```python
from build123d import *


with BuildPart() as f1:
    # F0 (on Front) → F1 (revolve)
    with BuildSketch(Plane.XZ):
        with BuildLine():
            Line((15.425971, 19.134293), (16, 0))
            Line((16, 0), (19, 0))
            Line((19, 0), (19.371627, 18.581355))
            ThreePointArc((19.371627, 18.581355), (19.209023, 19.949907), (18.678973, 21.22208))
            Line((18.678973, 21.22208), (17.092742, 23.910606))
            ThreePointArc((17.092742, 23.910606), (16.601144, 25.044324), (16.402601, 26.263982))
            Line((16.402601, 26.263982), (15.7, 45))
            Line((15.7, 45), (12.703474, 44.851139))
            Line((12.703474, 44.851139), (13.416649, 25.833132))
            ThreePointArc((13.416649, 25.833132), (13.518091, 25.00142), (13.756992, 24.198326))
            Line((13.756992, 24.198326), (15.084364, 20.806534))
            ThreePointArc((15.084364, 20.806534), (15.327049, 19.985097), (15.425971, 19.134293))
        make_face()
    revolve(axis=Axis((0, 0, 22.42557), (0, 0, 1)))


solid = f1.part
```
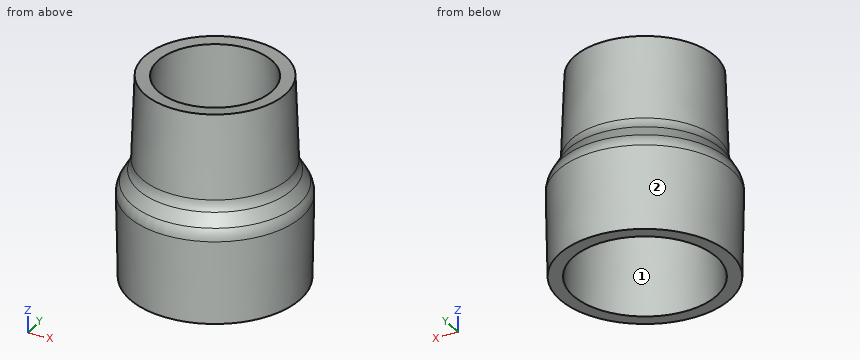
The listing builds one solid part. Answer for the finished solid, in the listing's coordinates (mm). Face numbers are marked on the shaded views. Give positions to 0.01 mm unless a question says otherwise; leave off trailing zeros. Order: outer loops, then holes, each group sorted by start corner. A loop starts at its lowest first (then second) coordinate and runs counter-clockwise, first axis right, second up. Notation, with made-up numbers: (24.5, 17.25) -> (47.5, 17.25) arc R5 ccw to (47.5, 24.25) -> close; hole circle Ø3 at (-33, -33). An arc over 180 degrees is marked (long way). Answer as a JSON object with one key per item and string values. Group by question number.
Item 1: Consider L1, parallel to Y at x = -4, z = 35; L2, parallel to X at y = 7.5, z = 6; L3, parallel to Y at x = 11, z = 31.5. Determine where each line is inside the solid, lowest interval first. Write a range as from..to.
Item 2: Flat-ended cylindrical pins translate along their axes: pin 1 (8 mm diameter, centred on x = 6, y = 6.5, fed in from +Z); pin 2 (10 mm diameter, centred on x = -12, z = 24.5, fed in from -Y); pin 3 (3 mm diameter, centred on y = -9, z = 35.5, fed in from +X). Find the tip coordinate at first contact, or state that the pin passes through.
Item 3: Determine the mould class of the marked faces 1 and 2 for opening direction X: pulls with the +X half, pulls with the -X half, needs draft (parallel to the pull), parting line crosses it, or undercut.
Item 4: The part is cut by section B-B on z = 32.5. Write down the section's boundary in (x, y), and give its area (3 significant figures).
Item 5: The part is cut by section A-A on z = 15. Write down the section's boundary in (x, y), and give its area (3 significant figures).
Result set:
{
 "1": {"L1": "-15.57..-12.45, 12.45..15.57", "L2": "-17.59..-13.93, 13.93..17.59", "L3": "-11.9..-7.3, 7.3..11.9"},
 "2": {"pin 1": "z = 44.86", "pin 2": "y = -16.81", "pin 3": "x = 14.2"},
 "3": {"face 1": "undercut", "face 2": "parting line crosses it"},
 "4": {"outline": "circle Ø32.34 at (0, 0); hole circle Ø26.33 at (0, 0)", "area": "277 mm²"},
 "5": {"outline": "circle Ø38.6 at (0, 0); hole circle Ø31.1 at (0, 0)", "area": "411 mm²"}
}
